from build123d import *

# Parameters (mm, degrees)
F1_DEPTH  = 7
F2_R      = 9.5
F3_DEPTH  = 10
F6_DEPTH  = 2.5
F4_R      = 5
F7_DEPTH  = 1
F8_W      = 6.5
F8_H      = 4.5
F9_DEPTH  = 2.5
F10_W     = 2
F10_H     = 1.5
F11_DEPTH = 1.5
F12_R     = 44.99999


# Not quite as in the source:
# - a fillet or chamfer is up to 0.001 mm smaller than in the source, because OpenCascade refuses the exact size


with BuildPart() as f1:
    # F0 (on Top) → F1 (new body)
    with BuildSketch(Plane.XY):
        with BuildLine():
            Line((-45, 70), (-45, 0))
            ThreePointArc((-45, 0), (0, -45), (45, 0))
            Line((45, 0), (45, 70))
            Line((45, 70), (-45, 70))
        make_face()
    extrude(amount=F1_DEPTH)

    # F2 (on face) → F3 (cut)
    with BuildSketch(Plane(origin=(0, 0, 0), x_dir=(1, 0, 0), z_dir=(0, 0, -1))):
        Circle(F2_R)
    extrude(amount=-F3_DEPTH, mode=Mode.SUBTRACT)

    # F5 (on face) → F6 (cut)
    with BuildSketch(Plane(origin=(0, 0, 0), x_dir=(1, 0, 0), z_dir=(0, 0, -1))):
        Polygon((20, 32.6008529611), (17.875, 33.8277222831), (15.625, 29.9306079661), (17.75, 28.7037386441), (17.75, 26.25), (22.25, 26.25), (22.25, 28.7037386441), (24.375, 29.9306079661), (22.125, 33.8277222831), align=None)
    extrude(amount=-F6_DEPTH, mode=Mode.SUBTRACT)

    # F4 (on face) → F7 (cut)
    with BuildSketch(Plane(origin=(0, 0, 0), x_dir=(1, 0, 0), z_dir=(0, 0, -1))):
        with Locations((0, -60)):
            Circle(F4_R)
    extrude(amount=-F7_DEPTH, mode=Mode.SUBTRACT)

    # F8 (on face) → F9 (cut)
    with BuildSketch(Plane(origin=(0, 0, 0), x_dir=(1, 0, 0), z_dir=(0, 0, -1))):
        with Locations((-20, 30)):
            Rectangle(F8_W, F8_H)
    extrude(amount=-F9_DEPTH, mode=Mode.SUBTRACT)

    # F10 (on face) → F11 (join)
    with BuildSketch(Plane(origin=(0, 0, 2.5), x_dir=(1, 0, 0), z_dir=(0, 0, -1))):
        with Locations((-20, 31.5)):
            Rectangle(F10_W, F10_H)
        with Locations((-20, 28.5)):
            Rectangle(F10_W, F10_H)
    extrude(amount=F11_DEPTH)

    # F12 (radius 45 in the source; OpenCascade refuses exactly that, so slightly less here)
    f12_edges = [f1.edges().sort_by_distance(p)[0] for p in [
        (-45, 70, 3.5),
        (45, 70, 3.5),
    ]]
    fillet(f12_edges, radius=F12_R)


solid = f1.part
Build history of the part. All positions in model axes, mm. A direction names the side the tool comes from. Coordinates: 2 decimals unless noted, no trailing zeros. Order: outer loops, then holes, each group sorted by start corner. A loop starts at its lowest first (then second) coordinate and runs counter-clockwise, first axis right, second up. Notation, with made-up numbers: (18.5, 65.25) - (71.5, 65.25) arc R21 ccw to (71.5, 71.25) - close; hole circle Ø4 at (-2, 31). An arc over 180 degrees is marked (long way). Write item = value, one per line. Start each with the question number.
1) 3-axis set-ups, long thin cutter, end or side, ignore diameter. For faces 4 (the face through (-1, 13, 7)), 5 (the face through (0, 60, 1)): which of +Z, -Z, +X, -X, +Y, -Y reach the whole face in a straight line?
2) Wall check: line 1 along X through (y, z) = (0, 4); line 2 along X through (y, z) = (60, 0.45); line 3 along Y through (x, z) = (-8, 0.75). Give the ranges that are in metal, low to high. Write a range as from..to.
3) Saw through at C-C on y = 60. Write the cut outline in (x, z), then the cut area to 3 significant figures.
4) Saw through at B-B on x = -3. Write the cut outline in (y, z).
5) Two-plate mould, pull along X, no slides. Class faces 1 (the face through (-20, -30, 2.5)), 2 (the face through (-45, 13, 3)), 3 (the face through (45, 12, 3)): pulls with the +X half, pulls with the -X half, needs draft (parallel to the pull), parting line crosses it, or undercut.
6) Saw through at D-D on x = -15. Write the cut outline in (y, z), then the cut area to 3 significant figures.
7) Flat gauge pins, fed straight in: pin 1 Ø2.5 at (y, z) = (-28, 1) entering from +X; pin 2 Ø2.5 at (y, z) = (-27.5, 1.5) entering from -X; pin 3 Ø1 at (y, z) = (34.5, 4.5) entering from +X. Where does each tip first touch, or does it go through?
From the geometry:
q1.face_4 = +Z, +X, -X, +Y, -Y
q1.face_5 = -Z
q2.line_1 = -45..-9.5, 9.5..45
q2.line_2 = -28.28..-5, 5..28.28
q2.line_3 = -44.28..-5.12, 5.12..69.28
q3.outline = (-28.28, 0) - (-5, 0) - (-5, 1) - (5, 1) - (5, 0) - (28.28, 0) - (28.28, 7) - (-28.28, 7) - close
q3.area = 386 mm^2
q4.outline = (-44.9, 0) - (-9.01, 0) - (-9.01, 7) - (-44.9, 7) - close; (9.01, 0) - (56, 0) - (56, 1) - (64, 1) - (64, 0) - (69.9, 0) - (69.9, 7) - (9.01, 7) - close
q5.face_1 = undercut
q5.face_2 = pulls with the -X half
q5.face_3 = pulls with the +X half
q6.outline = (-42.43, 0) - (67.43, 0) - (67.43, 7) - (-42.43, 7) - close
q6.area = 769 mm^2
q7.pin_1 = 36.19
q7.pin_2 = -36.55
q7.pin_3 = 44.09
